Read the model definition and answer for the solid it produces. Units are mm, in the model's axes. Face numbers are marked on the shaded views. A direction names the side the tool comes from. Coordinates: 2 decimals unless noted, no trailing zeros. Order: outer loops, then holes, each group sorted by start corner. A loop starts at its lowest first (then second) coordinate and runs counter-clockwise, first axis right, second up. Notation, with made-up numbers: (45, -30) - (85, -30) arc R24 cw to (85, 3) - close; hole circle Ø5 at (85.25, 84). An arc over 180 degrees is marked (long way). Answer as a JSON object with one key per item and string values. Group by question number.
from build123d import *

# Parameters (mm, degrees)
SKETCH1_W           = 10
SKETCH1_H           = 12
SKETCH1_R           = 3
BOSS_EXTRUDE1_DEPTH = 10
SKETCH2_R           = 1.5
CUT_EXTRUDE1_DEPTH  = 41.078048855
FILLET1_R           = 2


with BuildPart() as part:
    # Sketch1 → Boss-Extrude1 (new body)
    # profile 1 of 2: a face of its own
    with BuildSketch(Plane.XY):
        Rectangle(SKETCH1_W, SKETCH1_H)
        Circle(SKETCH1_R, mode=Mode.SUBTRACT)
    # profile 2 of 2: a face of its own
    with BuildSketch(Plane.XY):
        Polygon((-4, -6), (4, -6), (4, -37.5), (3, -37.5), (3, -33.5), (-3, -33.5), (-3, -37.5), (-4, -37.5), align=None)
    extrude(amount=BOSS_EXTRUDE1_DEPTH)

    # Sketch2 → Cut-Extrude1 (cut, through all)
    with BuildSketch(Plane.ZY.offset(5)):
        with Locations(Location((5, 0, 0), (0, 0, 270))):
            Circle(SKETCH2_R)
    extrude(amount=-CUT_EXTRUDE1_DEPTH, mode=Mode.SUBTRACT)

    # Fillet1
    # the kernel refuses this fillet: 2 mm, written as the material it adds along each edge
    with BuildSketch(Plane(origin=(4, -6, 0), x_dir=(1, 0, 0), z_dir=(0, 0, 1))) as fillet1_piece_1:
        with BuildLine():
            CenterArc((2, -1.732050808), FILLET1_R, 120, 60)
            Line((0, -1.732050808), (-0.04, -1.732050808))
            Line((-0.04, -1.732050808), (-0.04, 0))
            Line((-0.04, 0), (0, 0.04))
            ThreePointArc((0, 0.04), (0.5, 0.04), (0.98, 0.034641016))
            Line((0.98, 0.034641016), (1, 0))
        make_face()
    extrude(amount=10)
    with BuildSketch(Plane(origin=(-4, -6, 0), x_dir=(-1, 0, 0), z_dir=(0, 0, 1))) as fillet1_piece_2:
        with BuildLine():
            CenterArc((2, 1.732050808), FILLET1_R, 180, 60)
            Line((0, 1.732050808), (-0.04, 1.732050808))
            Line((-0.04, 1.732050808), (-0.04, 0))
            Line((-0.04, 0), (0, -0.04))
            ThreePointArc((0, -0.04), (0.5, -0.04), (0.98, -0.034641016))
            Line((0.98, -0.034641016), (1, 0))
        make_face()
    extrude(amount=10)


solid = part.part
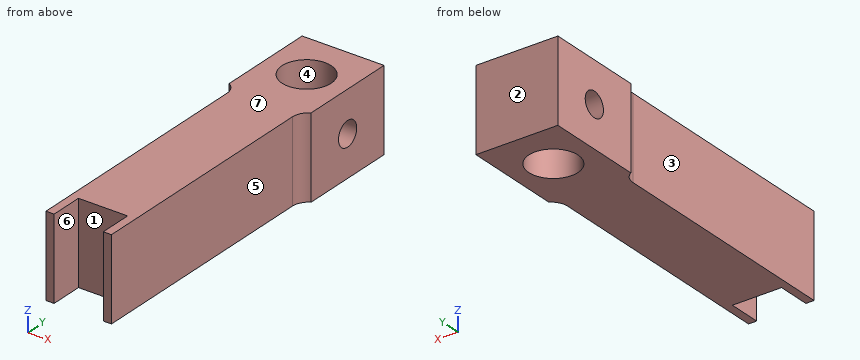
1. A cutting plane is placed at B-B on y = 0. Write down the section's boundary in (x, z).
2. For the marked faces 5, 6 and 7, determine the directions among +Z, -Z, +X, -X, +Y, -Y from which every point of the face is accessible in a straight line to the end or side of a thin tool.
3. Straight lines are drawn through the part: L1, parallel to X at y = 0, z = 2.25; L2, parallel to X at y = 1.5, z = 6; L3, parallel to Y at x = 3.3, z = 5. For each, find the intervals that lie inside material, in ascending order.
4. A cutting plane is placed at A-A on z = 5. Write down the section's boundary in (x, y), and give its area (3 significant figures).
5. Given pin 1 (2 mm diameter, centred on y = -36.5, z = 4.5, fed in from +X); pin 2 (3 mm diameter, centred on y = -36, z = 4, fed in from -X), each flat-ended and moving along its own axis, determine where each tip first touches the part or whether it passes through.
6. A cutting plane is placed at C-C on x = 0. Write down the section's boundary in (y, z), and give its area (3 significant figures).
7. A cutting plane is placed at D-D on z = 9. Write down the section's boundary in (x, y), and give its area (3 significant figures).
8. For a pull along X with two mould halves and no side action, classify the marked faces 1, 2, 3 and 4 as pulls with the +X half, pulls with the -X half, needs draft (parallel to the pull), parting line crosses it, or undercut.
Derived:
{
 "1": {"outline": "(-5, 0) - (-3, 0) - (-3, 3.5) - (-5, 3.5) - close; (-5, 6.5) - (-3, 6.5) - (-3, 10) - (-5, 10) - close; (3, 0) - (5, 0) - (5, 3.5) - (3, 3.5) - close; (3, 6.5) - (5, 6.5) - (5, 10) - (3, 10) - close"},
 "2": {"face 5": "+Z, -Z, +X, -Y", "face 6": "+Z, -Z, -Y", "face 7": "+Z, +X, -X, +Y, -Y"},
 "3": {"L1": "x = -5 to -3, 3 to 5", "L2": "x = -5 to -2.6, 2.6 to 5", "L3": "y = -37.5 to -1.5, 1.5 to 6"},
 "4": {"outline": "(-5, -6) arc R2 cw to (-4, -7.73) - (-4, -37.5) - (-3, -37.5) - (-3, -33.5) - (3, -33.5) - (3, -37.5) - (4, -37.5) - (4, -7.73) arc R2 cw to (5, -6) - (5, -1.5) - (2.6, -1.5) arc R3 cw to (-2.6, -1.5) - (-5, -1.5) - close; (-5, 1.5) - (-2.6, 1.5) arc R3 cw to (2.6, 1.5) - (5, 1.5) - (5, 6) - (-5, 6) - close", "area": "308 mm2"},
 "5": {"pin 1": "stops at x = 4", "pin 2": "stops at x = -4"},
 "6": {"outline": "(-33.5, 0) - (-3, 0) - (-3, 10) - (-33.5, 10) - close; (3, 0) - (6, 0) - (6, 10) - (3, 10) - close", "area": "335 mm2"},
 "7": {"outline": "(-5, -6) arc R2 cw to (-4, -7.73) - (-4, -37.5) - (-3, -37.5) - (-3, -33.5) - (3, -33.5) - (3, -37.5) - (4, -37.5) - (4, -7.73) arc R2 cw to (5, -6) - (5, 6) - (-5, 6) - close; hole circle Ø6 at (0, 0)", "area": "321 mm2"},
 "8": {"face 1": "undercut", "face 2": "needs draft", "face 3": "pulls with the -X half", "face 4": "undercut"}
}
